```python
from build123d import *

# Parameters (mm, degrees)
SKETCH1_W           = 130
SKETCH1_H           = 145.26
SKETCH1_R           = 3.6
SKETCH1_R_2         = 2.5
BOSS_EXTRUDE1_DEPTH = 9.4
SKETCH2_W           = 15
SKETCH2_H           = 30
CUT_EXTRUDE1_DEPTH  = 10.4
FILLET1_R           = 5


with BuildPart() as part:
    # Sketch1 → Boss-Extrude1 (new body)
    with BuildSketch(Plane.XY):
        with Locations((50, 62.63)):
            Rectangle(SKETCH1_W, SKETCH1_H)
        Circle(SKETCH1_R, mode=Mode.SUBTRACT)
        with Locations((0, 60.26)):
            Circle(SKETCH1_R_2, mode=Mode.SUBTRACT)
        with Locations((100, 60.26)):
            Circle(SKETCH1_R_2, mode=Mode.SUBTRACT)
        with Locations((100, 0)):
            Circle(SKETCH1_R, mode=Mode.SUBTRACT)
        with Locations((75.33, 82.555)):
            Circle(SKETCH1_R_2, mode=Mode.SUBTRACT)
        with Locations((105.33, 82.555)):
            Circle(SKETCH1_R_2, mode=Mode.SUBTRACT)
        with Locations((105.33, 122.635)):
            Circle(SKETCH1_R_2, mode=Mode.SUBTRACT)
        with Locations((75.33, 102.766411568)):
            Circle(SKETCH1_R_2, mode=Mode.SUBTRACT)
        with Locations((75.33, 122.766411568)):
            Circle(SKETCH1_R_2, mode=Mode.SUBTRACT)
    extrude(amount=BOSS_EXTRUDE1_DEPTH)

    # Sketch2 → Cut-Extrude1 (cut, through all)
    with BuildSketch(Plane(origin=(0, 0, 0), x_dir=(-1, 0, 0), z_dir=(0, 0, -1))):
        with Locations((-32.90754614, 102.570367495)):
            Rectangle(SKETCH2_W, SKETCH2_H)
    extrude(amount=-CUT_EXTRUDE1_DEPTH, mode=Mode.SUBTRACT)

    # Fillet1
    fillet1_edges = [part.edges().sort_by_distance(p)[0] for p in [
        (40.40754614, 87.570367495, 4.7),
        (40.40754614, 117.570367495, 4.7),
        (25.40754614, 117.570367495, 4.7),
        (25.40754614, 87.570367495, 4.7),
    ]]
    fillet(fillet1_edges, radius=FILLET1_R)


solid = part.part
```
Here's how the part is built. I have some questions about the finished solid (model axes, mm). A direction names the side the tool comes from. Round coordinates to 2 decimals unless told otherwise and drop trailing zeros. Write each loop counter-clockwise with the first axis right and the second up, starting at its lowest first coordinate (ties: lowest second). Pieces come first, ordered by that corner, then holes.
Q1. Will this pin go through, and if not, where does the flat tip stop? P1, Ø6.5, axis at x = 100, y = 0, coming from the +Z side.
Q2. If we section it at D-D on z = 1.5: Give the number of separate pieces and of enclosed holes in the cut face, plus the area to 3 significant figures.
Q3. If we section it at C-C on x = 75.33: Write out the boundary of the cut face in (y, z) (3 decimals).
Q4. If we mould it in two halves opening along Y, with no side actions, what happens to faces 1 (the cylindrical face through (73.487, 84.245, 4.634)), 2 (the cylindrical face through (-0.33, 62.74, 4.63)), 3 (the flat face through (49, 135.26, 5)), 4 (the flat face through (49, 64, 9.4))? For each: +Y half, -Y half, draft (parallel to the pull), parting line (faces both ways), or undercut.
Q5. If we section it at B-B on y = 0: Write out the boundary of the cut face in (x, z).
Q6. Please list where these lines run through material, in increasing order: probe 1 along X at (y, z) = (60, 3); probe 2 along Y at (x, z) = (75.33, 4) (3 decimals); probe 3 along Y at (x, z) = (0, 5.5).
Q7. If we section it at A-A on x = 100: Write out the boundary of the cut face in (y, z), plus the area to 3 significant figures.
Q8. Which directions (+Z, -Z, +X, -X, +Y, -Y) give clear straight access to the entire face, cutting with the end or side of a thin tool? Please do faces 5 (the flat face through (33, 87.57, 5)), 6 (the flat face through (-15, 62, 5)).
Answer below:
1. P1: passes through
2. separate pieces: 1
2. enclosed holes: 10
2. area: 18,200 mm2
3. outline: (-10, 0) - (80.055, 0) - (80.055, 9.4) - (-10, 9.4) - close; (85.055, 0) - (100.266, 0) - (100.266, 9.4) - (85.055, 9.4) - close; (105.266, 0) - (120.266, 0) - (120.266, 9.4) - (105.266, 9.4) - close; (125.266, 0) - (135.26, 0) - (135.26, 9.4) - (125.266, 9.4) - close
4. face 1: undercut
4. face 2: undercut
4. face 3: +Y half
4. face 4: draft
5. outline: (-15, 0) - (-3.6, 0) - (-3.6, 9.4) - (-15, 9.4) - close; (3.6, 0) - (96.4, 0) - (96.4, 9.4) - (3.6, 9.4) - close; (103.6, 0) - (115, 0) - (115, 9.4) - (103.6, 9.4) - close
6. probe 1: x = -15 to -2.49, 2.49 to 97.51, 102.49 to 115
6. probe 2: y = -10 to 80.055, 85.055 to 100.266, 105.266 to 120.266, 125.266 to 135.26
6. probe 3: y = -10 to -3.6, 3.6 to 57.76, 62.76 to 135.26
7. outline: (-10, 0) - (-3.6, 0) - (-3.6, 9.4) - (-10, 9.4) - close; (3.6, 0) - (57.76, 0) - (57.76, 9.4) - (3.6, 9.4) - close; (62.76, 0) - (135.26, 0) - (135.26, 9.4) - (62.76, 9.4) - close
7. area: 1,250 mm2
8. face 5: +Z, -Z
8. face 6: +Z, -Z, -X, +Y, -Y
